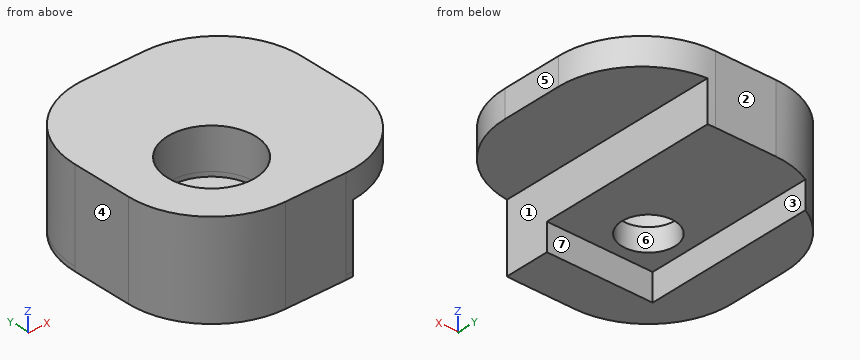
from build123d import *

# Parameters (mm, degrees)
ESBO_O3_W                = 7
ESBO_O3_H                = 12
ESBO_O3_R                = 1.75
RESSALTO_EXTRUS_O2_DEPTH = 2.7
ESBO_O4_W                = 7
ESBO_O4_H                = 12
ESBO_O4_R                = 1.75
RESSALTO_EXTRUS_O3_DEPTH = 2.1
ESBO_O5_W                = 2.1
ESBO_O5_H                = 12
RESSALTO_EXTRUS_O4_DEPTH = 5
RESSALTO_EXTRUS_O5_DEPTH = 3
ESBO_O7_W                = 4.8
ESBO_O7_H                = 15
RESSALTO_EXTRUS_O6_DEPTH = 3
ESBO_O8_R                = 2.9
CORTE_EXTRUS_O1_DEPTH    = 3
FILETE1_R                = 5.5
RESSALTO_EXTRUS_O7_DEPTH = 1.5
CORTE_EXTRUS_O4_DEPTH    = 6.3
CORTE_EXTRUS_O5_DEPTH    = 6.3
RESSALTO_EXTRUS_O8_DEPTH = 0.3
CORTE_EXTRUS_O6_DEPTH    = 0.3
ESBO_O17_R               = 2.9
CORTE_EXTRUS_O7_DEPTH    = 0.3


with BuildPart() as part:
    # Esboço3 → Ressalto-extrusão2 (new body)
    with BuildSketch(Plane.XY):
        with Locations((-3.5, 6)):
            Rectangle(ESBO_O3_W, ESBO_O3_H)
        with Locations((-2.5, 2.5)):
            Circle(ESBO_O3_R, mode=Mode.SUBTRACT)
    extrude(amount=RESSALTO_EXTRUS_O2_DEPTH)

    # Esboço4 → Ressalto-extrusão3 (add)
    with BuildSketch(Plane.XY.offset(2.7)):
        with Locations((-3.5, 6)):
            Rectangle(ESBO_O4_W, ESBO_O4_H)
        with Locations((-2.5, 2.5)):
            Circle(ESBO_O4_R, mode=Mode.SUBTRACT)
    extrude(amount=RESSALTO_EXTRUS_O3_DEPTH)

    # Esboço5 → Ressalto-extrusão4 (add)
    with BuildSketch(Plane.ZY.offset(7)):
        with Locations((3.75, 6)):
            Rectangle(ESBO_O5_W, ESBO_O5_H)
    extrude(amount=RESSALTO_EXTRUS_O4_DEPTH)

    # Esboço6 → Ressalto-extrusão5 (add)
    with BuildSketch(Plane.XZ):
        Polygon((-7, 0), (0, 0), (0, 4.8), (-12, 4.8), (-12, 2.7), (-7, 2.7), align=None)
    extrude(amount=RESSALTO_EXTRUS_O5_DEPTH)

    # Esboço7 → Ressalto-extrusão6 (add)
    with BuildSketch(Plane(origin=(0, 0, 0), x_dir=(0, 0, -1), z_dir=(1, 0, 0))):
        with Locations((-2.4, 4.5)):
            Rectangle(ESBO_O7_W, ESBO_O7_H)
    extrude(amount=RESSALTO_EXTRUS_O6_DEPTH)

    # Esboço8 → Corte-extrusão1 (cut)
    with BuildSketch(Plane.XY.offset(4.8)):
        with Locations((-2.5, 2.5)):
            Circle(ESBO_O8_R)
    extrude(amount=-CORTE_EXTRUS_O1_DEPTH, mode=Mode.SUBTRACT)

    # Filete1
    filete1_edges = [part.edges().sort_by_distance(p)[0] for p in [
        (3, -3, 2.4),
    ]]
    fillet(filete1_edges, radius=FILETE1_R)

    # Esboço10 → Ressalto-extrusão7 (add)
    with BuildSketch(Plane(origin=(0, 0, 0), x_dir=(-1, 0, 0), z_dir=(0, 0, -1))):
        with BuildLine():
            Line((7, 0), (0, 0))
            Line((0, 0), (0, 12))
            Line((0, 12), (-3, 12))
            Line((-3, 12), (-3, 2.5))
            ThreePointArc((-3, 2.5), (-1.389087297, -1.389087297), (2.5, -3))
            Line((2.5, -3), (7, -3))
            Line((7, -3), (7, 0))
        make_face()
    extrude(amount=RESSALTO_EXTRUS_O7_DEPTH)

    # Esboço14 → Corte-extrusão4 (cut)
    with BuildSketch(Plane.XY.offset(4.8)):
        with BuildLine():
            Line((-12, 12), (-12, 6.5))
            ThreePointArc((-12, 6.5), (-10.389087297, 10.389087297), (-6.5, 12))
            Line((-6.5, 12), (-12, 12))
        make_face()
        with BuildLine():
            ThreePointArc((-2.5, 12), (1.389087297, 10.389087297), (3, 6.5))
            Line((3, 6.5), (3, 12))
            Line((3, 12), (-2.5, 12))
        make_face()
    extrude(amount=-CORTE_EXTRUS_O4_DEPTH, mode=Mode.SUBTRACT)

    # Esboço13 → Corte-extrusão5 (cut)
    with BuildSketch(Plane.XY.offset(4.8)):
        with BuildLine():
            Line((-12, -3), (-6.5, -3))
            ThreePointArc((-6.5, -3), (-10.389087297, -1.389087297), (-12, 2.5))
            Line((-12, 2.5), (-12, -3))
        make_face()
    extrude(amount=-CORTE_EXTRUS_O5_DEPTH, mode=Mode.SUBTRACT)

    # Esboço15 → Ressalto-extrusão8 (add)
    with BuildSketch(Plane(origin=(0, 0, -1.5), x_dir=(-1, 0, 0), z_dir=(0, 0, -1))):
        with BuildLine():
            Line((2.5, -3), (6.5, -3))
            ThreePointArc((6.5, -3), (6.750259203, -2.994303444), (7, -2.977225575))
            Line((7, -2.977225575), (7, 0))
            Line((7, 0), (0, 0))
            Line((0, 0), (0, 11.398979486))
            ThreePointArc((0, 11.398979486), (-2.19041576, 9.372281323), (-3, 6.5))
            Line((-3, 6.5), (-3, 2.5))
            ThreePointArc((-3, 2.5), (-1.389087297, -1.389087297), (2.5, -3))
        make_face()
    extrude(amount=RESSALTO_EXTRUS_O8_DEPTH)


with BuildPart() as body_2:
    # Espelhar3: mirrored copy
    add(part.part.mirror(Plane(origin=(4, 0, 0), x_dir=(0, 0, 1), z_dir=(1, 0, 0))))

    # Esboço16 → Corte-extrusão6 (cut)
    with BuildSketch(Plane.XY.offset(4.8)):
        with BuildLine():
            Line((20, 2.5), (20, 6.5))
            ThreePointArc((20, 6.5), (18.389087297, 10.389087297), (14.5, 12))
            Line((14.5, 12), (10.5, 12))
            ThreePointArc((10.5, 12), (6.610912703, 10.389087297), (5, 6.5))
            Line((5, 6.5), (5, 2.5))
            ThreePointArc((5, 2.5), (6.610912703, -1.389087297), (10.5, -3))
            Line((10.5, -3), (14.5, -3))
            ThreePointArc((14.5, -3), (18.389087297, -1.389087297), (20, 2.5))
        make_face()
    extrude(amount=-CORTE_EXTRUS_O6_DEPTH, mode=Mode.SUBTRACT)

    # Esboço17 → Corte-extrusão7 (cut)
    with BuildSketch(Plane.XY.offset(1.8)):
        with Locations((10.5, 2.5)):
            Circle(ESBO_O17_R)
    extrude(amount=-CORTE_EXTRUS_O7_DEPTH, mode=Mode.SUBTRACT)


solid = body_2.part
Geometry check sheet. Reference: the model listing, model coordinates, mm. Face numbers are marked on the shaded views. A direction names the side the tool comes from. Give positions to 0.01 mm unless a question says otherwise; leave off trailing zeros. Loops run counter-clockwise (first coordinate to the right, second up) from the corner with the lowest first, then second, coordinate; pieces in that order, holes last.
(1) Section check C-C on x = 14. Record the cut outline in (y, z).
From the geometry:
outline: (-3, -1.8) - (0, -1.8) - (0, 0) - (12, 0) - (12, 4.5) - (-3, 4.5) - close
(2) Section check B-B on y = 1.75. Record the cut outline in (x, z), then the cut area to 3 significant figures.
From the geometry:
outline: (5.05, -1.8) - (8, -1.8) - (8, 0) - (8.92, 0) - (8.92, 1.5) - (7.7, 1.5) - (7.7, 4.5) - (5.05, 4.5) - close; (12.08, 0) - (15, 0) - (15, 2.7) - (19.95, 2.7) - (19.95, 4.5) - (13.3, 4.5) - (13.3, 1.5) - (12.08, 1.5) - close
area: 37.4 mm2
(3) Depth check by flat-ended pin: pin 1 Ø3 at (x, y) = (10.5, 3.5) entering from +Z; pin 2 Ø2.5 at (x, y) = (16.5, 5) entering from -Z; pin 3 Ø1 at (y, z) = (2.5, 0) entering from +X. Enter the tip coordinate at first touch or a pass-through.
From the geometry:
pin 1: stops at z = 1.5
pin 2: stops at z = 2.7
pin 3: stops at x = 15
(4) Section check A-A on z = 3. Record the cut outline in (x, y).
From the geometry:
outline: (5, 2.5) arc R5.5 ccw to (10.5, -3) - (14.5, -3) arc R5.5 ccw to (20, 2.5) - (20, 6.5) arc R5.5 ccw to (14.5, 12) - (10.5, 12) arc R5.5 ccw to (5, 6.5) - close; hole circle Ø5.8 at (10.5, 2.5)
(5) Section check D-D on z = -0.75. Record the cut outline in (x, y).
From the geometry:
outline: (5, 2.5) arc R5.5 ccw to (10.5, -3) - (14.5, -3) arc R5.5 ccw to (15, -2.98) - (15, 0) - (8, 0) - (8, 11.4) arc R5.5 ccw to (5, 6.5) - close
(6) Release check for a two-part mould opening along X. For the marked faces 4, 5, 6 and 7 record: released by +X, released by -X, zero draft, split by the parting line, or undercut.
From the geometry:
face 4: released by -X
face 5: released by +X
face 6: undercut
face 7: zero draft
(7) Set-up check for the marked faces 1, 2 and 3: record each of +Z, -Z, +X, -X, +Y, -Y from which the full face is reachable in a straight line by a thin tool's end or side.
From the geometry:
face 1: -Z, +X, +Y, -Y
face 2: +Z, -Z, +X, -X, +Y
face 3: -Z, +X, +Y
(8) Thickness scan on L1, parallel to X at y = 2.5, z = 1.7; L2, parallel to Y at x = 10.5, z = 1.75; L3, parallel to Y at x = 10.5, z = 0.3. Record the ranges inside material, lowest first.
From the geometry:
L1: x = 5 to 7.6, 13.4 to 15
L2: y = -3 to -0.4, 5.4 to 12
L3: y = -3 to 0.75, 4.25 to 12
